```python
from build123d import *

# Parameters (mm, degrees)
HOLES_R            = 3.25
CUT_EXTRUDE2_DEPTH = 121.915154753
SKETCH9_R          = 1.8
PROBE_HOLE_DEPTH   = 57
FILLET1_R          = 10
FILLET2_R          = 0.5
FILLET3_R          = 1.2


with BuildPart() as part:
    # Cross_section → Revolve 2 (revolve)
    with BuildSketch(Plane.XY, mode=Mode.PRIVATE) as revolve_2_sk:
        with BuildLine():
            Line((21.032889293, 6.834), (39.942176945, 12.978))
            Line((39.942176945, 12.978), (39.942176945, 27.978))
            Line((39.942176945, 27.978), (7.796597981, 43.2))
            Line((7.796597981, 43.2), (-36.7, 43.2))
            Line((-36.7, 43.2), (-36.7, 60))
            Line((-36.7, 60), (-46.2, 60))
            Line((-46.2, 60), (-46.2, 31))
            Line((-46.2, 31), (-46.7, 31))
            Line((-46.7, 31), (-46.7, 25))
            Line((-46.7, 25), (0, 25))
            ThreePointArc((0, 25), (4.5, 23.794228634), (7.794228634, 20.5))
            Line((7.794228634, 20.5), (13.238660659, 11.334))
            ThreePointArc((13.238660659, 11.334), (16.532889293, 8.039771366), (21.032889293, 6.834))
        make_face()
    revolve(revolve_2_sk.sketch.rotate(Axis((0, 0, 0), (1, 0, 0)), 90), axis=Axis((0, 0, 0), (1, 0, 0)))

    # holes → Cut-Extrude2 (cut, through all)
    with BuildSketch(Plane.ZY.offset(46.2)):
        with Locations((0, 51.6)):
            Circle(HOLES_R)
        with Locations((30.329719018, 41.74527691)):
            Circle(HOLES_R)
        with Locations((49.074516241, 15.94527691)):
            Circle(HOLES_R)
        with Locations((49.074516241, -15.94527691)):
            Circle(HOLES_R)
        with Locations((30.329719018, -41.74527691)):
            Circle(HOLES_R)
        with Locations((0, -51.6)):
            Circle(HOLES_R)
        with Locations((-30.329719018, -41.74527691)):
            Circle(HOLES_R)
        with Locations((-49.074516241, -15.94527691)):
            Circle(HOLES_R)
        with Locations((-49.074516241, 15.94527691)):
            Circle(HOLES_R)
        with Locations((-30.329719018, 41.74527691)):
            Circle(HOLES_R)
    extrude(amount=-CUT_EXTRUDE2_DEPTH, mode=Mode.SUBTRACT)

    # Sketch9 → probe_hole (cut)
    with BuildSketch(Plane(origin=(0, 0, 0), x_dir=(1, 0, 0), z_dir=(0, -0.587785252292477, 0.8090169943749446))):
        with Locations(Location((-23.35, 0, 0), (0, 0, 270))):
            Circle(SKETCH9_R)
    extrude(amount=-PROBE_HOLE_DEPTH, mode=Mode.SUBTRACT)

    # Fillet1
    fillet1_edges = [part.edges().sort_by_distance(p)[0] for p in [
        (7.796597981, 0, -43.2),
    ]]
    fillet(fillet1_edges, radius=FILLET1_R)

    # Fillet2
    fillet2_edges = [part.edges().sort_by_distance(p)[0] for p in [
        (-36.7, 0, -43.2),
    ]]
    fillet(fillet2_edges, radius=FILLET2_R)

    # Fillet3
    fillet3_edges = [part.edges().sort_by_distance(p)[0] for p in [
        (21.032889293, 0, -6.834),
    ]]
    fillet(fillet3_edges, radius=FILLET3_R)


solid = part.part
```
Check sheet for the modelled part. Datum: model origin and axes. Units: mm. A direction names the side the tool comes from. Round coordinates to 2 decimals unless told otherwise and drop trailing zeros. Loops run counter-clockwise (first coordinate to the right, second up) from the corner with the lowest first, then second, coordinate; pieces in that order, holes last. Notation, with made-up numbers: (-7, 0.25) -> (46, 0.25) arc R21 ccw to (46, 22.25) -> close; hole circle Ø8 at (-30, 49). An arc over 180 degrees is marked (long way). Write item = value, one per line. Start each with the question number.
1) Sectioned sample at A-A, the plane y = 50. Record the cut outline in (x, z).
2) Thickness scan on probe 1 along X at (y, z) = (31, -40); probe 2 along Z at (x, y) = (-18, 20.5); probe 3 along Z at (x, y) = (-23, 4). Record the ranges inside material, lowest first.
3) Set-up check for faces 4 (the flat face through (39.942, 6, -12)), 5 (the flat face through (-46.2, 26, 26)): record each of +Z, -Z, +X, -X, +Y, -Y from which the full face is reachable in a straight line by a thin tool's end or side.
4) Sectioned sample at D-D, the plane y = -51.6. Record the cut outline in (x, z), plus the area to 3 significant figures.
5) Sectioned sample at B-B, the plane x = -5. Record the cut outline in (y, z), plus the area to 3 significant figures.
6) Sectioned sample at C-C, the plane z = 0. State how many separate pieces and enclosed holes the cut face has, plus the area to 3 significant figures.
7) Release check for a two-part mould opening along Y. For faces 1 (the cylindrical face through (-46.454, -30.736, -4.036)), 2 (the flat face through (-36.7, 17.5, 40.3)), 3 (the cylindrical face through (-41.52, 39.77, -32.91)) record: released by +Y, released by -Y, zero draft, split by the parting line, or undercut.
8) Gauge pin test, flat ends, axial feed: pin 1 Ø3 at (y, z) = (-34, 25) entering from -X; pin 2 Ø8.5 at (y, z) = (-15.95, -49.07) entering from +X; pin 3 Ø5 at (x, y) = (21.5, -25) entering from -Z. Record the tip position at first contact, or that the pin passes through.
Results are:
q1.outline = (-46.2, -33.17) -> (-36.7, -33.17) -> (-36.7, -2.83) -> (-46.2, -2.83) -> close; (-46.2, 2.83) -> (-36.7, 2.83) -> (-36.7, 33.17) -> (-46.2, 33.17) -> close
q2.probe_1 = -46.2 to -36.7
q2.probe_2 = -38.03 to -14.31, 14.31 to 38.03
q2.probe_3 = -43.01 to -24.68, 24.68 to 43.01
q3.face_4 = +Z, -Z, +X, +Y, -Y
q3.face_5 = -X
q4.outline = (-46.2, -30.62) -> (-36.7, -30.62) -> (-36.7, -3.25) -> (-46.2, -3.25) -> close; (-46.2, 3.25) -> (-36.7, 3.25) -> (-36.7, 30.62) -> (-46.2, 30.62) -> close
q4.area = 520 mm^2
q5.outline = circle Ø86.4 at (0, 0); hole circle Ø50 at (0, 0)
q5.area = 3,900 mm^2
q6.separate_pieces = 4
q6.enclosed_holes = 0
q6.area = 3,800 mm^2
q7.face_1 = split by the parting line
q7.face_2 = zero draft
q7.face_3 = undercut
q8.pin_1 = -46.2
q8.pin_2 = -36.7
q8.pin_3 = -29.52
